Solid Edge part; units mm, degrees
sketch "Sketch1" plane through (0, 0, 0) normal (0, 0, 1) x (1, 0, 0)
  circle A0 centre (0, 0) radius 15
extrude "ExtrudedProtrusion_1" add sketch "Sketch1" along normal blind 10
sketch "Sketch2" plane through (8.5, 0, 0) normal (-1, 0, 0) x (0, -1, 0)
  line L0 (3.35, 5) -> (3.35, 10)
  line L1 (-3.35, 10) -> (3.35, 10)
  line L2 (-3.35, 5) -> (-3.35, 10)
  line L3 (-3.35, 5) -> (-1.675, 2.0988)
  line L4 (-1.675, 2.0988) -> (1.675, 2.0988)
  line L5 (1.675, 2.0988) -> (3.35, 5)
  circle A0 centre (0, 5) radius 1.65
extrude "ExtrudedCutout_1" cut sketch "Sketch2" along normal mid plane 3.2
mirror "Mirror1" about plane through (0, 0, 0) normal (-1, 0, 0) of "ExtrudedCutout_1"
sketch "Sketch3" plane through (8.5, 0, 0) normal (-1, 0, 0) x (0, -1, 0)
  circle A0 centre (0, 5) radius 1.65
extrude "Cutout1" cut sketch "Sketch3" against normal through all and the other way through all
sketch "Sketch4" plane through (0, 0, 10) normal (0, 0, 1) x (-1, 0, 0)
  circle A0 centre (-3, 0) radius 2
  circle A1 centre (3, 0) radius 2
extrude "ExtrudedCutout_3" cut sketch "Sketch4" against normal blind 6
chamfer "Chamfer_3" distance 1 angle 45 2 edges at (-1, 0, 10) (5, 0, 10)
Here's how the part is built. I have some questions about the finished solid (model axes, mm). A direction names the side the tool comes from. Coordinates: 2 decimals unless noted, no trailing zeros. Loops run counter-clockwise (first coordinate to the right, second up) from the corner with the lowest first, then second, coordinate; pieces in that order, holes last. Notation, with made-up numbers: M 55,-4.75 L 81,-4.75 A18 ccw 81,15.25 Z; hole C 24,-7.75 d6. An arc over 180 degrees is marked long. One line per item, written item: value.
1. On a 3-axis mill with a long thin cutter (end or side, diameter ignored), from which of +Z, -Z, +X, -X, +Y, -Y can I reach the whole of each face in a straight line? I mean faces 3 (the flat face through (0, 0, 0)), 4 (the flat face through (-9, 3.35, 8)). Say none if no direction works.
Geometry says:
face 3: -Z, +X, -X, +Y, -Y
face 4: +Z
2. Please list where these lines run through material, in increasing order: probe 1 along Z at (x, y) = (-13, 0); probe 2 along Z at (x, y) = (-0.5, 0); probe 3 along Y at (x, z) = (12.7, 5).
Geometry says:
probe 1: z = 0 to 3.35, 6.65 to 10
probe 2: z = 0 to 3.35, 6.65 to 9.5
probe 3: y = -7.98 to -1.65, 1.65 to 7.98
3. Imagine slicing it at B-B (z = 3). List the corners of the cut face in (x, y) for me.
Geometry says:
outline: C 0,0 d30; hole M -10.1,-2.2 L -6.9,-2.2 L -6.9,2.2 L -10.1,2.2 Z; hole M 6.9,-2.2 L 10.1,-2.2 L 10.1,2.2 L 6.9,2.2 Z
4. Thinking about a two-plate mould opening in Y: for faces 1 (the flat face through (0, -3, 10)), 2 (the flat face through (-10.1, 0, 7)), which applies, +Y half, -Y half, draft (parallel to the pull), parting line (faces both ways), or undercut?
Geometry says:
face 1: draft
face 2: undercut
5. Imagine slicing it at D-D (y = 0). State how many separate pieces and enclosed holes the cut face has, and give its area (3 significant figures).
Geometry says:
separate pieces: 6
enclosed holes: 0
area: 143 mm2
6. Imagine slicing it at A-A (z = 8.5). List the corners of the cut face in (x, y) for me, and give its area (3 significant figures).
Geometry says:
outline: C 0,0 d30; hole M -10.1,-3.35 L -6.9,-3.35 L -6.9,3.35 L -10.1,3.35 Z; hole C -3,0 d4; hole C 3,0 d4; hole M 6.9,-3.35 L 10.1,-3.35 L 10.1,3.35 L 6.9,3.35 Z
area: 639 mm2
7. Imagine slicing it at C-C (x = -8.5). List the corners of the cut face in (y, z) for me (3 decimals), and give its area (3 significant figures).
Geometry says:
outline: M -12.359,0 L 12.359,0 L 12.359,10 L 3.35,10 L 3.35,5 L 1.675,2.099 L -1.675,2.099 L -3.35,5 L -3.35,10 L -12.359,10 Z
area: 199 mm2
8. Will these pins go through, and if not, where does the flat tip stop? pin 1 Ø1 at (x, z) = (6.5, 2) entering from +Y; pin 2 Ø2 at (y, z) = (-1, 5.5) entering from -X; pin 3 Ø1.6 at (x, z) = (8, 6.5) entering from -Y; pin 4 Ø5.5 at (y, z) = (1.5, 5.5) entering from +X.
Geometry says:
pin 1: stops at y = 13.75
pin 2: stops at x = -14.98
pin 3: stops at y = -13.16
pin 4: stops at x = 15
